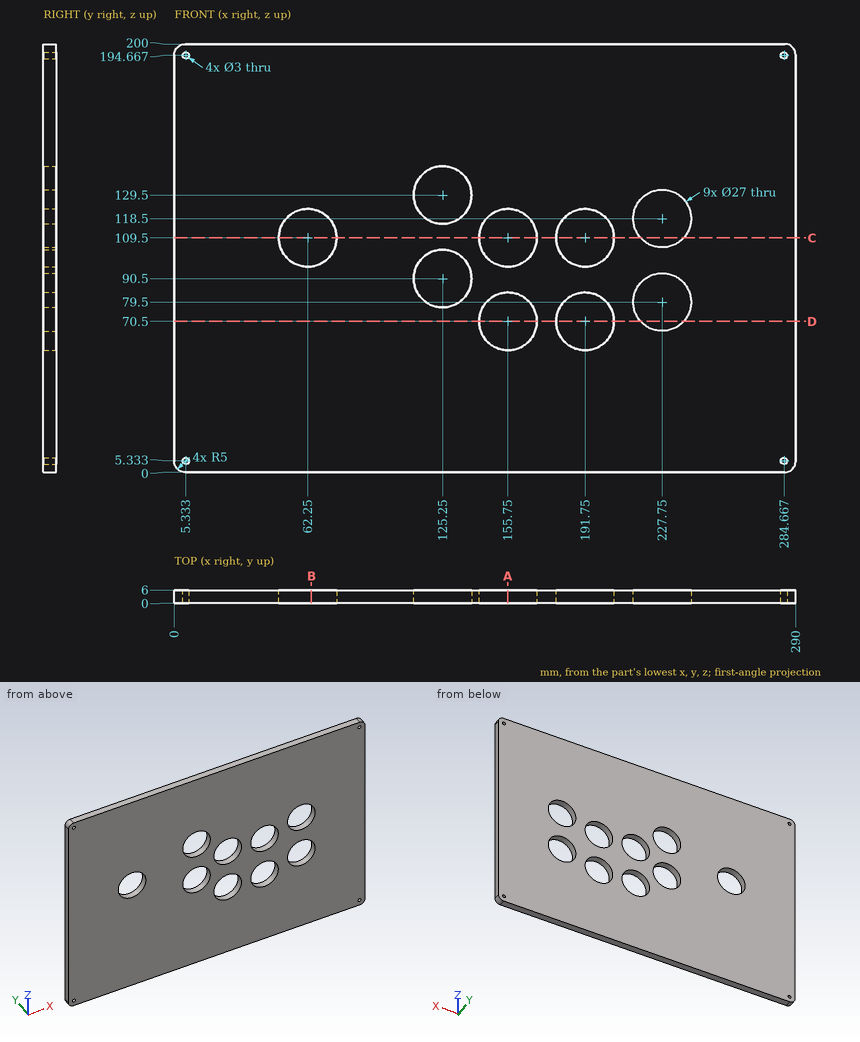
Could you check a few things on this drawing? It's one solid part, dimensions in mm from its lowest x, y, z. Give positions to 0.01 mm unless a question says otherwise; leave off trailing zeros. Order: outer loops, then holes, each group sorted by start corner. A loop starts at its lowest first (then second) coordinate and runs counter-clockwise, first axis right, second up. Notation, with made-up numbers: M 47,-40 L 64,-40 A9 ccw 64,-28 Z; hole C -5.75,88 d7. An arc over 180 degrees is marked long. Use one line per item in the form item = value. Start each with the question number.
Item 1: If we section it at A-A (x = 155.75): Write out the boundary of the cut face in (y, z), then the cut area to 3 significant figures.
Item 2: If we section it at D-D (z = 70.5): Write out the boundary of the cut face in (x, y).
Item 3: Will this pin go through, and if not, where does the flat tip stop? pin 1 Ø21.5 at (x, z) = (125.25, 90.5) entering from +Y.
Item 4: If we section it at C-C (z = 109.5): Write out the boundary of the cut face in (x, y).
Item 5: If we section it at B-B (x = 64): Write out the boundary of the cut face in (y, z), then the cut area to 3 significant figures.
Item 6: If I drill on line 1 along Z through (x, y) = (227.75, 3.4); line 2 along Z through (x, y) = (125.25, 3.05); line 3 along X through (y, z) = (4.3, 70.5), over which ranges is the centre line in solid material (lowest first)?
Outcome:
q1.outline = M 0,0 L 6,0 L 6,57 L 0,57 Z; M 0,84 L 6,84 L 6,96 L 0,96 Z; M 0,123 L 6,123 L 6,200 L 0,200 Z
q1.area = 876 mm2
q2.outline = M 0,0 L 142.25,0 L 142.25,6 L 0,6 Z; M 169.25,0 L 178.25,0 L 178.25,6 L 169.25,6 Z; M 205.25,0 L 217.69,0 L 217.69,6 L 205.25,6 Z; M 237.81,0 L 290,0 L 290,6 L 237.81,6 Z
q3.pin_1 = through
q4.outline = M 0,0 L 48.75,0 L 48.75,6 L 0,6 Z; M 75.75,0 L 142.25,0 L 142.25,6 L 75.75,6 Z; M 169.25,0 L 178.25,0 L 178.25,6 L 169.25,6 Z; M 205.25,0 L 217.69,0 L 217.69,6 L 205.25,6 Z; M 237.81,0 L 290,0 L 290,6 L 237.81,6 Z
q5.outline = M 0,0 L 6,0 L 6,96.11 L 0,96.11 Z; M 0,122.89 L 6,122.89 L 6,200 L 0,200 Z
q5.area = 1,040 mm2
q6.line_1 = 0 to 66, 93 to 105, 132 to 200
q6.line_2 = 0 to 77, 104 to 116, 143 to 200
q6.line_3 = 0 to 142.25, 169.25 to 178.25, 205.25 to 217.69, 237.81 to 290
